```python
from build123d import *

# Parameters (mm, degrees)
CROQUIS1_W              = 64
CROQUIS1_H              = 44
CROQUIS1_R              = 5
CROQUIS1_R_2            = 3.5
SALIENTE_EXTRUIR1_DEPTH = 3
CROQUIS3_W              = 60
CROQUIS3_H              = 40
CROQUIS3_W_2            = 56
CROQUIS3_H_2            = 36
SALIENTE_EXTRUIR2_DEPTH = 3


with BuildPart() as part:
    # Croquis1 → Saliente-Extruir1 (new body)
    with BuildSketch(Plane.XY):
        with Locations((-32, 22)):
            Rectangle(CROQUIS1_W, CROQUIS1_H)
        with Locations((-52, 34)):
            Circle(CROQUIS1_R, mode=Mode.SUBTRACT)
        with Locations((-52, 10)):
            Circle(CROQUIS1_R, mode=Mode.SUBTRACT)
        with Locations((-20, 22)):
            Circle(CROQUIS1_R_2, mode=Mode.SUBTRACT)
        with Locations((-52, 22)):
            Circle(CROQUIS1_R, mode=Mode.SUBTRACT)
    extrude(amount=SALIENTE_EXTRUIR1_DEPTH)

    # Croquis3 → Saliente-Extruir2 (add)
    with BuildSketch(Plane.XY.offset(3)):
        with Locations((-32, 22)):
            Rectangle(CROQUIS3_W, CROQUIS3_H)
        with Locations((-32, 22)):
            Rectangle(CROQUIS3_W_2, CROQUIS3_H_2, mode=Mode.SUBTRACT)
    extrude(amount=SALIENTE_EXTRUIR2_DEPTH)


solid = part.part
```
Can you work these out from the model? Positions are in its coordinate system, mm. A direction names the side the tool comes from. Round coordinates to 2 decimals unless told otherwise and drop trailing zeros. Loops run counter-clockwise (first coordinate to the right, second up) from the corner with the lowest first, then second, coordinate; pieces in that order, holes last.
Item 1: Please list where these lines run through material, in increasing order: L1, parallel to Y at x = -52, z = 1.7; L2, parallel to Y at x = -20, z = 1.65; L3, parallel to X at y = 23, z = 3.7.
Item 2: Suppose I cut it at C-C, the plane x = -9. Write out the boundary of the cut face in (y, z), then the cut area to 3 significant figures.
Item 3: Which directions (+Z, -Z, +X, -X, +Y, -Y) give clear straight access to the entire face, cutting with the end or side of a thin tool? Please do faces 1 (the flat face through (-32, 2, 4)), 2 (the flat face through (-32, 40, 4)), 3 (the flat face through (-62, 22, 4)), 4 (the flat face through (-2, 22, 4)).
Item 4: Suppose I cut it at D-D, the plane x = -19. Write out the boundary of the cut face in (y, z).
Item 5: Will these pins go through, and if not, where does the flat tip stop? pin 1 Ø2.5 at (x, z) = (-25.5, 5) entering from -Y; pin 2 Ø10 at (x, y) = (-12.5, 19) entering from +Z; pin 3 Ø8 at (x, y) = (-52, 22) entering from +Z; pin 4 Ø1.5 at (x, z) = (-46, 4) entering from +Y.
Item 6: Suppose I cut it at A-A, the plane y = 22. Write out the boundary of the cut face in (x, z).
Item 7: Suppose I cut it at B-B, the plane z = 1.2. Write out the boundary of the cut face in (x, y), then the cut area to 3 significant figures.
Item 8: If we mould it in two halves opening along X, with no side actions, what happens to faces 5 (the flat face through (-4, 22, 4)), 6 (the flat face through (-32, 22, 0)), 7 (the flat face through (0, 22, 1))? For each: +X half, -X half, draft (parallel to the pull), parting line (faces both ways), or undercut.
Reported:
1. L1: y = 0 to 5, 15 to 17, 27 to 29, 39 to 44
1. L2: y = 0 to 18.5, 25.5 to 44
1. L3: x = -62 to -60, -4 to -2
2. outline: (0, 0) - (44, 0) - (44, 3) - (42, 3) - (42, 6) - (40, 6) - (40, 3) - (4, 3) - (4, 6) - (2, 6) - (2, 3) - (0, 3) - close
2. area: 144 mm2
3. face 1: +Z, +X, -X, -Y
3. face 2: +Z
3. face 3: +Z, -X, +Y, -Y
3. face 4: +Z, +X, +Y, -Y
4. outline: (0, 0) - (18.65, 0) - (18.65, 3) - (4, 3) - (4, 6) - (2, 6) - (2, 3) - (0, 3) - close; (25.35, 0) - (44, 0) - (44, 3) - (42, 3) - (42, 6) - (40, 6) - (40, 3) - (25.35, 3) - close
5. pin 1: stops at y = 2
5. pin 2: stops at z = 3
5. pin 3: passes through
5. pin 4: stops at y = 42
6. outline: (-64, 0) - (-57, 0) - (-57, 3) - (-60, 3) - (-60, 6) - (-62, 6) - (-62, 3) - (-64, 3) - close; (-47, 0) - (-23.5, 0) - (-23.5, 3) - (-47, 3) - close; (-16.5, 0) - (0, 0) - (0, 3) - (-2, 3) - (-2, 6) - (-4, 6) - (-4, 3) - (-16.5, 3) - close
7. outline: (-64, 0) - (0, 0) - (0, 44) - (-64, 44) - close; hole circle Ø10 at (-52, 10); hole circle Ø10 at (-52, 22); hole circle Ø10 at (-52, 34); hole circle Ø7 at (-20, 22)
7. area: 2,540 mm2
8. face 5: undercut
8. face 6: draft
8. face 7: +X half
